For this review, take the finished solid that the model builds, in its own axes (mm). Face numbers are marked on the shaded views. A direction names the side the tool comes from. Round coordinates to 2 decimals unless told otherwise and drop trailing zeros. Write each loop counter-clockwise with the first axis right and the second up, starting at its lowest first coordinate (ties: lowest second). Pieces come first, ordered by that corner, then holes. Notation, with made-up numbers: (-13, 66) -> (21, 66) arc R34 ccw to (21, 97) -> close; hole circle Ø7 at (12, 50). An arc over 180 degrees is marked (long way). Answer as CSV lines item,"result". Start each with the question number.
Item 1: Wall thickness on probe 1 along Y at (x, z) = (0, 1.7) (3 decimals); probe 2 along Y at (x, z) = (0, 5.75); probe 3 along X at (y, z) = (-0.5, 6.25): over which ranges is each line inside the solid? List them lowest first. Write a range as from..to.
Item 2: For pin 1 Ø5 at (x, y) = (0, 0) entering from +Z; pin 2 Ø1.5 at (y, z) = (1, 5.5) entering from -X; pin 3 Ø1.5 at (x, z) = (-6, 5) entering from +Y, all flat-tipped, find the tip position at first contact; note any pin that passes through.
Item 3: Take a section at B-B on z = 4.25. Count the separate pieces of the cut face and the enclosed holes in it, then the cut area to 3 significant figures.
Item 4: Machinability: for the marked faces 1, 2 and 3, which of the approach directions +Z, -Z, +X, -X, +Y, -Y give a long, thin tool a straight path to every point of the face, cutting with its end or side? Answer none if there is none.
Item 5: Mouldability with a two-part tool opening along Y and no side actions: class the marked faces 4 and 5 as +Y half, -Y half, draft (parallel to the pull), parting line (faces both ways), or undercut.
Item 6: Take a section at A-A on y = 0. Give the boundary of the cut face in (x, z) (1 decimal), then the cut area to 3 significant figures.
```python
from build123d import *

# Parameters (mm, degrees)
F0_R     = 25.447764
F1_DEPTH = 7.62
F0_R_2   = 1.905
F2_DEPTH = 2.54
F4_R     = 1.8415


with BuildPart() as f1:
    # F0 (on Top) → F1 (new body)
    with BuildSketch(Plane.XY):
        Circle(F0_R)
        with BuildLine():
            ThreePointArc((-15.074386, -17.193977), (-21.736663, -7.098412), (-22.316716, 4.983389))
            ThreePointArc((-22.316716, 4.983389), (-21.955689, 5.476274), (-21.348665, 5.545541))
            Line((-21.348665, 5.545541), (-9.361943, 1.852396))
            ThreePointArc((-9.361943, 1.852396), (-8.947922, 1.540235), (-8.829496, 1.035425))
            ThreePointArc((-8.829496, 1.035425), (-8.445105, -2.777104), (-6.491723, -6.073684))
            ThreePointArc((-6.491723, -6.073684), (-6.287275, -6.553007), (-6.438668, -7.051635))
            Line((-6.438668, -7.051635), (-13.962558, -17.078354))
            ThreePointArc((-13.962558, -17.078354), (-14.493227, -17.378917), (-15.074386, -17.193977))
        make_face(mode=Mode.SUBTRACT)
        with BuildLine():
            Line((-11.892139, -18.55065), (-4.316171, -8.45453))
            ThreePointArc((-4.316171, -8.45453), (-3.90732, -8.176769), (-3.41405, -8.208311))
            ThreePointArc((-3.41405, -8.208311), (0.194774, -8.887866), (3.770364, -8.050867))
            ThreePointArc((3.770364, -8.050867), (4.289406, -8.004544), (4.716846, -8.302613))
            Line((4.716846, -8.302613), (11.927812, -18.556683))
            ThreePointArc((11.927812, -18.556683), (12.049678, -19.154259), (11.694203, -19.649824))
            ThreePointArc((11.694203, -19.649824), (0.013149, -22.866346), (-11.671596, -19.66326))
            ThreePointArc((-11.671596, -19.66326), (-12.030108, -19.156162), (-11.892139, -18.55065))
        make_face(mode=Mode.SUBTRACT)
        with BuildLine():
            Line((13.967844, -17.042562), (6.706966, -6.717516))
            ThreePointArc((6.706966, -6.717516), (6.569141, -6.242843), (6.751568, -5.783462))
            ThreePointArc((6.751568, -5.783462), (8.503922, -2.591411), (8.829496, 1.035425))
            ThreePointArc((8.829496, 1.035425), (8.947922, 1.540235), (9.361943, 1.852395))
            Line((9.361943, 1.852395), (21.348665, 5.545541))
            ThreePointArc((21.348665, 5.545541), (21.955689, 5.476274), (22.316716, 4.983389))
            ThreePointArc((22.316716, 4.983389), (21.740741, -7.085911), (15.09415, -17.176629))
            ThreePointArc((15.09415, -17.176629), (14.501085, -17.360892), (13.967844, -17.042562))
        make_face(mode=Mode.SUBTRACT)
        with BuildLine():
            ThreePointArc((-1.27, 9.435681), (-1.439174, 8.956931), (-1.871579, 8.690759))
            ThreePointArc((-1.871579, 8.690759), (-5.121211, 7.266725), (-7.555153, 4.68527))
            ThreePointArc((-7.555153, 4.68527), (-7.935438, 4.373286), (-8.427105, 4.358645))
            Line((-8.427105, 4.358645), (-20.498814, 8.077976))
            ThreePointArc((-20.498814, 8.077976), (-20.966736, 8.487792), (-20.973365, 9.10977))
            ThreePointArc((-20.973365, 9.10977), (-13.407682, 18.523068), (-2.102049, 22.769527))
            ThreePointArc((-2.102049, 22.769527), (-1.518548, 22.57379), (-1.27, 22.010753))
            Line((-1.27, 22.010753), (-1.27, 9.435681))
        make_face(mode=Mode.SUBTRACT)
        Polygon((6.379143, -3.683), (0, -7.366), (-6.379143, -3.683), (-6.379143, 3.683), (0, 7.366), (6.379143, 3.683), align=None, mode=Mode.SUBTRACT)
        with BuildLine():
            Line((1.27, 9.435681), (1.27, 22.010753))
            ThreePointArc((1.27, 22.010753), (1.518548, 22.57379), (2.102049, 22.769527))
            ThreePointArc((2.102049, 22.769527), (13.407682, 18.523068), (20.973365, 9.10977))
            ThreePointArc((20.973365, 9.10977), (20.966736, 8.487792), (20.498814, 8.077976))
            Line((20.498814, 8.077976), (8.427105, 4.358645))
            ThreePointArc((8.427105, 4.358645), (7.935438, 4.373285), (7.555154, 4.68527))
            ThreePointArc((7.555154, 4.68527), (5.121212, 7.266725), (1.871579, 8.690759))
            ThreePointArc((1.871579, 8.690759), (1.439174, 8.956931), (1.27, 9.435681))
        make_face(mode=Mode.SUBTRACT)
    extrude(amount=F1_DEPTH)

    # F0 (on Top) → F2 (join)
    with BuildSketch(Plane.XY):
        Polygon((-6.379143, -3.683), (0, -7.366), (6.379143, -3.683), (6.379143, 3.683), (0, 7.366), (-6.379143, 3.683), align=None)
        Circle(F0_R_2, mode=Mode.SUBTRACT)
    extrude(amount=F2_DEPTH)


with BuildPart() as f5:
    # F4 (on Front) → F5 (revolve)
    with BuildSketch(Plane.XZ):
        with Locations((25.4, 3.81)):
            Circle(F4_R)
    revolve(axis=Axis((0, 0, -1.325227), (0, 0, -1)))


with BuildPart() as f1_1:
    add(f1.part)

    # F6: cut F5
    add(f5.part, mode=Mode.SUBTRACT)


solid = f1_1.part
```
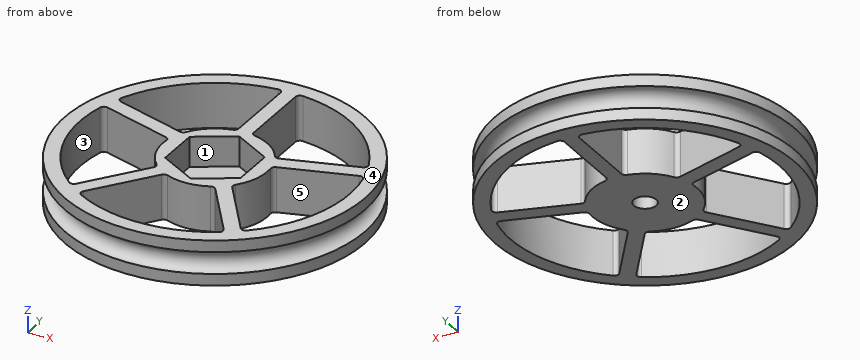
Output values:
1,probe 1,"y = -25.448..-22.866, -8.89..-1.905, 1.905..25.448"
1,probe 2,"y = -25.45..-22.87, -8.89..-7.37, 7.37..25.45"
1,probe 3,"x = -25.44..-22.86, -8.88..-6.38, 6.38..8.88, 22.86..25.44"
2,pin 1,"stops at z = 2.54"
2,pin 2,"stops at x = -25.45"
2,pin 3,"stops at y = 24.82"
3,separate pieces,"1"
3,enclosed holes,"6"
3,area,"400 mm^2"
4,face 1,"+Z"
4,face 2,"-Z, +X, -X, +Y, -Y"
4,face 3,"+Z, -Z"
5,face 4,"draft"
5,face 5,"undercut"
6,outline,"(-25.4, 0) -> (-22.9, 0) -> (-22.9, 7.6) -> (-25.4, 7.6) -> (-25.4, 5.7) arc R1.8 cw (long way) to (-25.4, 2) -> close; (-8.9, 0) -> (-1.9, 0) -> (-1.9, 2.5) -> (-6.4, 2.5) -> (-6.4, 7.6) -> (-8.9, 7.6) -> close; (1.9, 0) -> (8.9, 0) -> (8.9, 7.6) -> (6.4, 7.6) -> (6.4, 2.5) -> (1.9, 2.5) -> close; (22.9, 0) -> (25.4, 0) -> (25.4, 2) arc R1.8 cw (long way) to (25.4, 5.7) -> (25.4, 7.6) -> (22.9, 7.6) -> close"
6,area,"89.3 mm^2"
